```python
from build123d import *

# Parameters (mm, degrees)
F1_DEPTH = 1.5


with BuildPart() as f1:
    # F0 (on Front) → F1 (new body, symmetric)
    with BuildSketch(Plane.XZ):
        Polygon((12.7, 18), (5.8595971335, 36.7938524157), (3.1559015792, 35.4938407428), (0.9892154577, 40), (0, 40), (-0.9892154577, 40), (-3.1559015792, 35.4938407428), (-5.8595971335, 36.7938524157), (-12.7, 18), (-12.7, 5), (-15.7, 5), (-15.7, -5), (-12.7, -5), (-12.7, -33.66908), (-2.7, -43.66908), (0, -43.66908), (2.7, -43.66908), (12.7, -33.66908), (12.7, -5), (15.7, -5), (15.7, 5), (12.7, 5), align=None)
        Polygon((6.7, -31.1837986258), (2.2147186258, -35.66908), (-2.2147186258, -35.66908), (-6.7, -31.1837986258), (-6.7, -5), (-6.7, 5), (-6.7, 16.9420381157), (-3.7671417253, 25), (3.7671417253, 25), (6.7, 16.9420381157), (6.7, 5.483887788), (6.7, -4.516112212), align=None, mode=Mode.SUBTRACT)
    extrude(amount=F1_DEPTH, both=True)


solid = f1.part
```
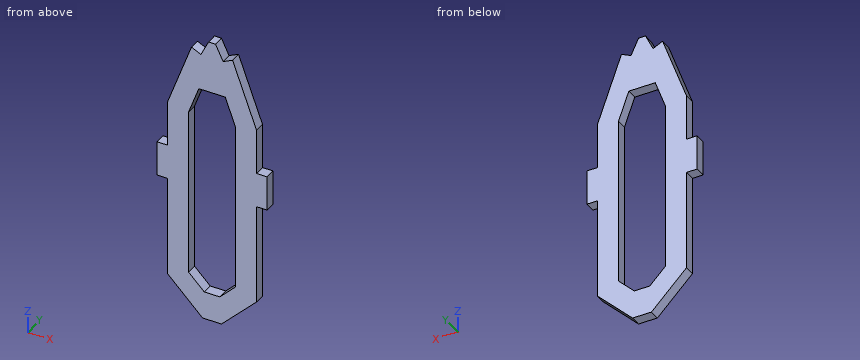
Here's how the part is built. I have some questions about the finished solid (model axes, mm). Give positions to 0.01 mm unless a question says otherwise; leave off trailing zeros. Order: outer loops, then holes, each group sorted by start corner. A loop starts at its lowest first (then second) coordinate and runs counter-clockwise, first axis right, second up. Notation, with made-up numbers: (30.25, 76) -> (45.25, 76) arc R20 cw to (45.25, 107) -> close; hole circle Ø2 at (-11.75, 29). An arc over 180 degrees is marked (long way). Use CSV: the item, a comma, the result in double quotes. Start each with the question number.
Item 1: Suppose I cut it at D-D (x = -7.5). List the corners of the cut face in (y, z) for me.
Item 2: I'm going to push flat-ended pins straight in: P1, Ø0.9, axis at y = 0.5, z = 11, coming from the +X side; P2, Ø1.5, axis at x = -14, y = 0, coming from the +Z side; P3, Ø1, axis at x = 2.5, y = 0, coming from the +Z side. Where does each tip first touch, or does it pass through?
Item 3: If I drill on probe 1 along X at (y, z) = (-0.75, 15); probe 2 along Z at (x, y) = (1, -0.7); probe 3 along Z at (x, y) = (-3, 0), over which ranges is the centre line in solid material (lowest first)? Write a range as [from, to].
Item 4: Suppose I cut it at B-B (z = -25.5). List the corners of the cut face in (x, y) for me.
Item 5: Suppose I cut it at A-A (y = 0.5). List the corners of the cut face in (x, z) for me, and give its area (3 significant figures).
Item 6: Suppose I cut it at C-C (x = 5). List the corners of the cut face in (y, z) for me.
Answer block:
1,outline,"(-1.5, -38.87) -> (1.5, -38.87) -> (1.5, 32.29) -> (-1.5, 32.29) -> close"
2,P1,"stops at x = 12.7"
2,P2,"stops at z = 5"
2,P3,"stops at z = 37.9"
3,probe 1,"x = [-12.7, -6.7], [6.7, 12.7]"
3,probe 2,"z = [-43.67, -35.67], [25, 39.98]"
3,probe 3,"z = [-43.37, -34.88], [25, 35.82]"
4,outline,"(-12.7, -1.5) -> (-6.7, -1.5) -> (-6.7, 1.5) -> (-12.7, 1.5) -> close; (6.7, -1.5) -> (12.7, -1.5) -> (12.7, 1.5) -> (6.7, 1.5) -> close"
5,outline,"(-15.7, -5) -> (-12.7, -5) -> (-12.7, -33.67) -> (-2.7, -43.67) -> (2.7, -43.67) -> (12.7, -33.67) -> (12.7, -5) -> (15.7, -5) -> (15.7, 5) -> (12.7, 5) -> (12.7, 18) -> (5.86, 36.79) -> (3.16, 35.49) -> (0.99, 40) -> (-0.99, 40) -> (-3.16, 35.49) -> (-5.86, 36.79) -> (-12.7, 18) -> (-12.7, 5) -> (-15.7, 5) -> close; hole (-6.7, -31.18) -> (-2.21, -35.67) -> (2.21, -35.67) -> (6.7, -31.18) -> (6.7, 16.94) -> (3.77, 25) -> (-3.77, 25) -> (-6.7, 16.94) -> close"
5,area,"1,110 mm^2"
6,outline,"(-1.5, -41.37) -> (1.5, -41.37) -> (1.5, -32.88) -> (-1.5, -32.88) -> close; (-1.5, 21.61) -> (1.5, 21.61) -> (1.5, 36.38) -> (-1.5, 36.38) -> close"
